Read the model definition and answer for the solid it produces. Units are mm, in the model's axes. Face numbers are marked on the shaded views. A direction names the side the tool comes from. Give positions to 0.01 mm unless a question says otherwise; leave off trailing zeros. Loops run counter-clockwise (first coordinate to the right, second up) from the corner with the lowest first, then second, coordinate; pieces in that order, holes last. Notation, with made-up numbers: (-16.75, 57) - (21.25, 57) arc R13 cw to (21.25, 73) - close; hole circle Ø11 at (-29, 68). An arc over 180 degrees is marked (long way). Use a Markdown table: item, result. Add a question column.
Item 1: A cutting plane is placed at A-A (z = 6). Determine the outline of the cut face in (x, y).
Item 2: Each of these flat-tipped pins is pushed along its axis until it touches: P1, Ø6.5, axis at x = -0.5, y = 22, coming from the +Z side; P2, Ø3.5, axis at x = -0.15, y = 21, coming from the +Z side; P3, Ø6.5, axis at y = 14, z = 24, coming from the +X side; P4, Ø6, axis at y = 10.5, z = -10.5, coming from the +X side. Where does it stop, or does it pass through?
Item 3: Which of the six approach directions +Z, -Z, +X, -X, +Y, -Y give full straight-line access (tool end or side, diameter ignored) to the marked faces 4, 5 and 6?
Item 4: Consider probe 1 along X at (y, z) = (23.5, 0); probe 2 along X at (y, z) = (18, -12.5); probe 3 along Z at (x, y) = (8, 3). Determine where each line is inside the solid, lowest interval first. Write a range as [from, to].
Item 5: For a pull along Z with two mould halves and no side action, classify the marked faces 1, 2 and 3 as +Z half, -Z half, draft (parallel to the pull), parting line (faces both ways), or undercut.
Item 6: A cutting plane is placed at C-C (y = 13). Determine the outline of the cut face in (x, z), plus the area to 3 significant figures.
Item 7: A cutting plane is placed at B-B (x = 0). Determine the outline of the cut face in (y, z).
Item 8: A cutting plane is placed at D-D (z = 22.5). Determine the outline of the cut face in (x, y), plus the area to 3 significant figures.
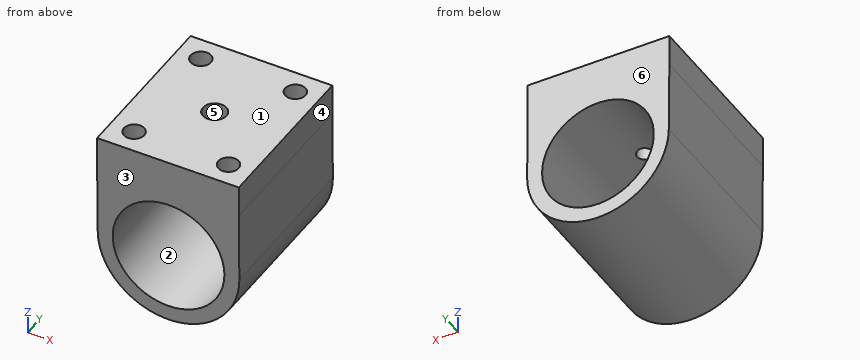
Autodesk Fusion 360 part; units mm, degrees
sketch "Skizze1" plane through (0, 0, 0) normal (0, 1, 0) x (1, 0, 0)
  circle A0 centre (0, 0) radius 14.2
  line L0 (-18.1535, -18) -> (17.8465, -18)
  line L1 (17.8465, -18) -> (17.8465, -26)
  line L2 (17.8465, -26) -> (-18.1535, -26)
  line L3 (-18.1535, -26) -> (-18.1535, -18)
  line L4 (-18.1535, -18) -> (17.8465, -26) construction
  line L5 (17.8465, -18) -> (-18.1535, -26) construction
  circle A1 centre (0, 0) radius 18
  line L6 (-18.1535, -18) -> (-17.9994, 0.1529)
  line L7 (17.8465, -18) -> (17.9993, -0.1542)
  point P0 (-0.1535, -22)
  dimension "d1" = 28.4
  dimension "d2" = 36
  dimension "d3" = 8
  dimension "d4" = 36
extrude "Extrusion1" add sketch "Skizze1" along normal blind 42
sketch "Skizze3" plane through (0, 0, 26) normal (0, 0, 1) x (1, 0, 0)
  line L0 (-18.1535, 0) -> (17.8465, 0)
  line L1 (17.8465, 0) -> (17.8465, 42)
  line L2 (17.8465, 42) -> (-18.1535, 42)
  line L3 (-18.1535, 42) -> (-18.1535, 0)
  circle A0 centre (-12.1535, 36) radius 2.6
  circle A1 centre (11.8465, 36) radius 2.6
  circle A2 centre (-12.1535, 6) radius 2.6
  circle A3 centre (11.8465, 6) radius 2.6
  dimension "d7" = 5.2
  dimension "d8" = 5.2
  dimension "d9" = 5.2
  dimension "d10" = 5.2
  dimension "d11" = 24
  dimension "d12" = 24
  dimension "d13" = 30
  dimension "d14" = 30
  dimension "d15" = 6
  dimension "d16" = 6
  dimension "d17" = 6
extrude "Extrusion2" cut sketch "Skizze3" against normal blind 14 contours A0 | A1 | A2 | A3
sketch "Skizze4" plane through (0, 0, 26) normal (0, 0, 1) x (1, 0, 0)
  circle A0 centre (-12.1535, 6) radius 2.6
  circle A1 centre (11.8465, 36) radius 2.6
  circle A2 centre (-12.1535, 36) radius 2.6
  circle A3 centre (11.8465, 6) radius 2.6
  line L0 (-18.1535, 0) -> (17.8465, 0)
  line L1 (17.8465, 0) -> (17.8465, 42)
  line L2 (17.8465, 42) -> (-18.1535, 42)
  line L3 (-18.1535, 42) -> (-18.1535, 0)
  line L4 (-18.1535, 0) -> (17.8465, 42) construction
  line L5 (17.8465, 0) -> (-18.1535, 42) construction
  circle A4 centre (-0.1535, 21) radius 3
  circle A5 centre (-0.1535, 21) radius 2.05
  dimension "d20" = 6
  dimension "d21" = 4.1
extrude "Extrusion3" cut sketch "Skizze4" against normal blind 16 contours A5
extrude "Extrusion4" cut sketch "Skizze4" against normal blind 5.5 contours A4
equation "d8 = d7"
equation "d9 = d7"
equation "d10 = d7"
equation "d15 = ( ( 36 - 24 ) / 2 ) * 1 mm"
equation "d16 = ( ( 42 - 30 ) / 2 ) * 1 mm"
equation "d17 = d15"
Geometry says:
| question | item | result |
|---|---|---|
| 1 | outline | (-18.05, 0) - (-12.87, 0) - (-12.87, 42) - (-18.05, 42) - close; (12.87, 0) - (17.95, 0) - (17.95, 42) - (12.87, 42) - close |
| 2 | P1 | z = 26 |
| 2 | P2 | z = -14.07 |
| 2 | P3 | x = 17.85 |
| 2 | P4 | x = 16.36 |
| 3 | face 4 | +Z, +X, +Y, -Y |
| 3 | face 5 | +Z |
| 3 | face 6 | +Z, -Z, +X, -X, +Y |
| 4 | probe 1 | [-18, -14.2], [14.2, 18] |
| 4 | probe 2 | [-12.95, -6.74], [6.74, 12.95] |
| 4 | probe 3 | [-16.12, -11.73], [11.73, 26] |
| 5 | face 1 | +Z half |
| 5 | face 2 | undercut |
| 5 | face 3 | draft |
| 6 | outline | (-18.15, 18) - (-18, -0.15) arc R18 ccw to (18, 0.15) - (17.85, 18) - (17.85, 26) - (-18.15, 26) - close; hole circle Ø28.4 at (0, 0) |
| 6 | area | 811 mm² |
| 7 | outline | (0, -18) - (42, -18) - (42, -14.2) - (0, -14.2) - close; (0, 14.2) - (18.96, 14.2) - (18.96, 20.5) - (18, 20.5) - (18, 26) - (0, 26) - close; (23.04, 14.2) - (42, 14.2) - (42, 26) - (24, 26) - (24, 20.5) - (23.04, 20.5) - close |
| 8 | outline | (-18.15, 0) - (17.85, 0) - (17.85, 42) - (-18.15, 42) - close; hole circle Ø5.2 at (-12.15, 6); hole circle Ø5.2 at (-12.15, 36); hole circle Ø6 at (-0.15, 21); hole circle Ø5.2 at (11.85, 6); hole circle Ø5.2 at (11.85, 36) |
| 8 | area | 1,400 mm² |
